Input: dimensioned drawing with shaded views. Units: mm. Origin: part minimum x, y, z. Give positions to 0.01 mm unless a question says otherwise; leave off trailing zeros. Write each loop counter-clockwise with the first axis right and the second up, starting at its lowest first coordinate (ties: lowest second). Pieces come first, ordered by that corner, then holes.
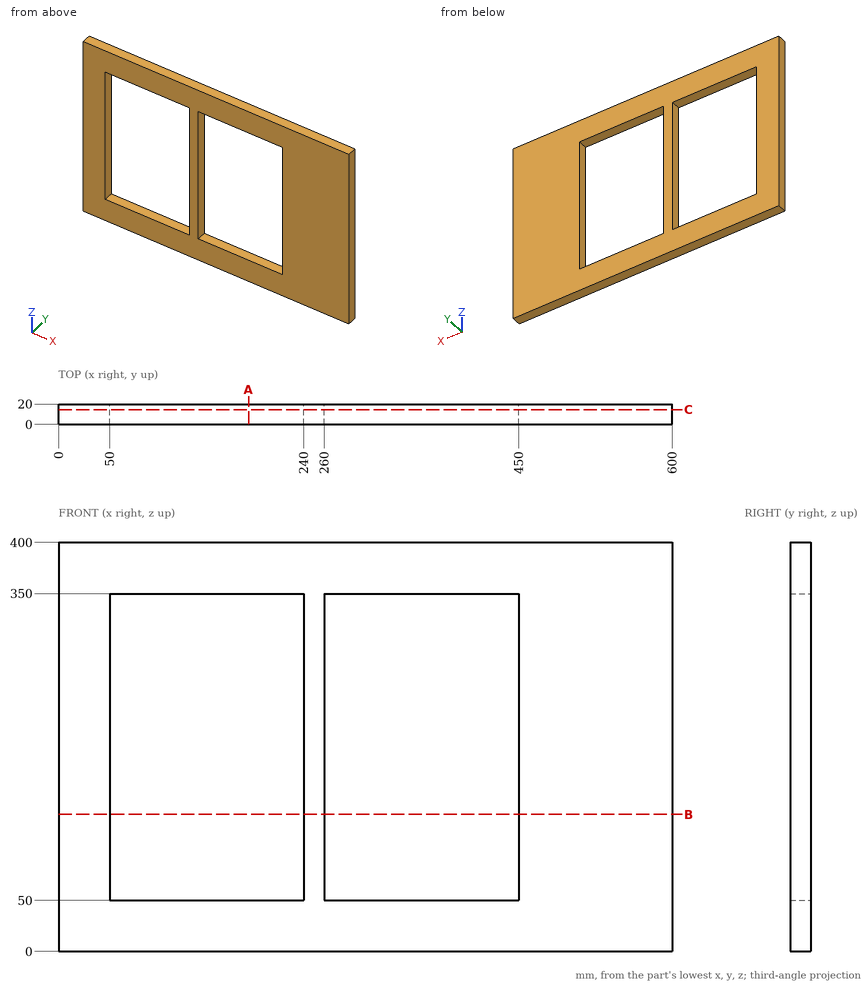
Item 1: Section A-A (x = 186). Return loops of the section in (y, z).
Item 2: Section C-C (y = 14.5). Return loops of the section in (x, z).
Item 3: Ray query, line 1 (X direction, y = 18.25, z = 325); line 2 (Z direction, x = 354, y = 14.5). Return the intervals inside material, ascending.
Item 4: Section B-B (z = 134). Return loops of the section in (x, y), and give its area (3 significant figures).
Solved:
1. outline: (0, 0) - (20, 0) - (20, 50) - (0, 50) - close; (0, 350) - (20, 350) - (20, 400) - (0, 400) - close
2. outline: (0, 0) - (600, 0) - (600, 400) - (0, 400) - close; hole (50, 50) - (240, 50) - (240, 350) - (50, 350) - close; hole (260, 50) - (450, 50) - (450, 350) - (260, 350) - close
3. line 1: x = 0 to 50, 240 to 260, 450 to 600
3. line 2: z = 0 to 50, 350 to 400
4. outline: (0, 0) - (50, 0) - (50, 20) - (0, 20) - close; (240, 0) - (260, 0) - (260, 20) - (240, 20) - close; (450, 0) - (600, 0) - (600, 20) - (450, 20) - close
4. area: 4,400 mm2
